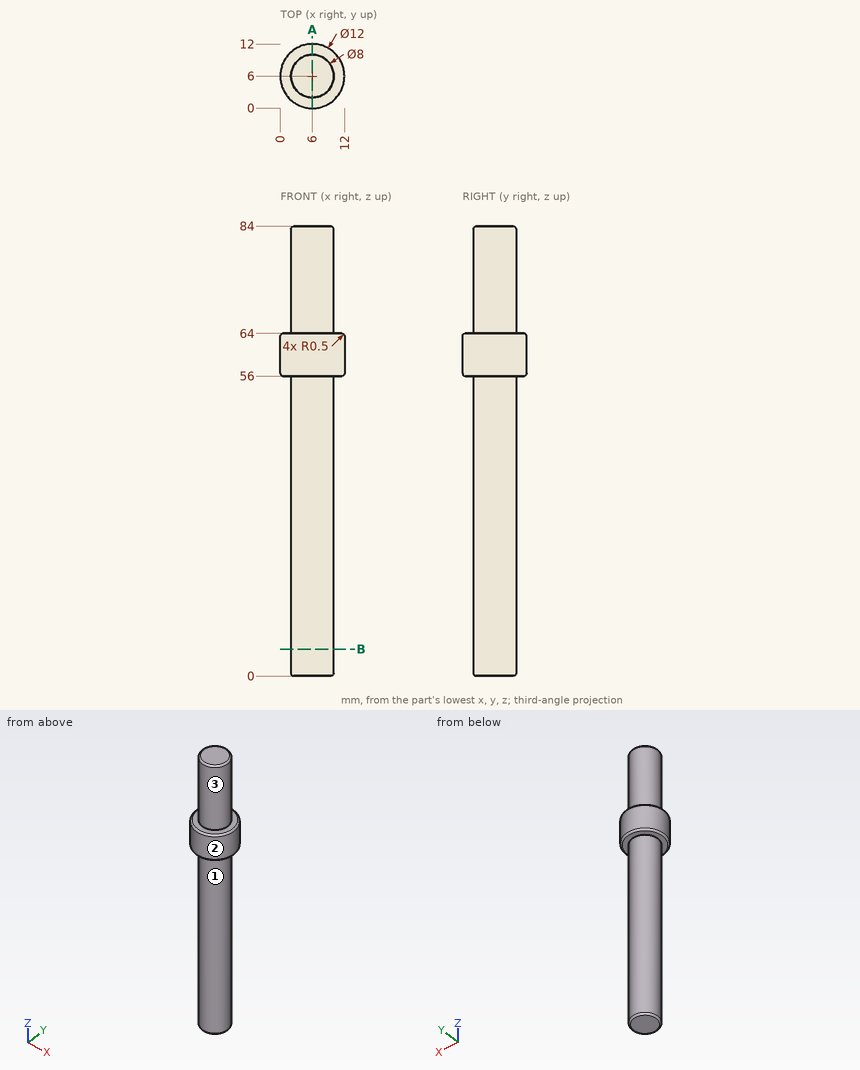
For this review, use the dimensioned drawing (mm, ordinates from the lowest corner) and the shaded views. A direction names the side the tool comes from. Give positions to 0.01 mm unless a question says otherwise; leave off trailing zeros. Order: outer loops, then holes, each group sorted by start corner. A loop starts at its lowest first (then second) coordinate and runs counter-clockwise, first axis right, second up.
1) Take a section at A-A (x = 6). Give the boundary of the cut face in (y, z), then the cut area to 3 significant figures.
2) Insertion check: pin 1 (5 mm diameter, centred on y = 6.5, z = 48, fed in from -X); pin 2 (2 mm diameter, centred on y = 10.5, z = 30, fed in from -X); pin 3 (4 mm diameter, centred on y = 1.5, z = 20, fed in from +X). Each pin has a flat end and moves straight along its axis. Give the tip position at first contact, or say it passes through.
3) Take a section at B-B (z = 5). Give the boundary of the cut face in (x, y).
4) For the marked faces 1, 2 and 3, list the 3-axis set-ups (+Z, -Z, +X, -X, +Y, -Y) from which the entire face can be reached by the end or side of a thin tool; tool diameter is ignored.
5) Wall thickness on line 1 (Z direction, x = 10.5, y = 4.25); line 2 (Z direction, x = 4, y = 3); line 3 (Y direction, x = 6, z = 74.5): over which ranges is each line inside the solid? List them lowest first.
Derived:
1. outline: (0, 56.5) arc R0.5 ccw to (0.5, 56) - (2, 56) - (2, 0.5) arc R0.5 ccw to (2.5, 0) - (9.5, 0) arc R0.5 ccw to (10, 0.5) - (10, 56) - (11.5, 56) arc R0.5 ccw to (12, 56.5) - (12, 63.5) arc R0.5 ccw to (11.5, 64) - (10, 64) - (10, 83.5) arc R0.5 ccw to (9.5, 84) - (2.5, 84) arc R0.5 ccw to (2, 83.5) - (2, 64) - (0.5, 64) arc R0.5 ccw to (0, 63.5) - close
1. area: 704 mm2
2. pin 1: stops at x = 2
2. pin 2: stops at x = 4.06
2. pin 3: stops at x = 9.12
3. outline: circle Ø8 at (6, 6)
4. face 1: -Z
4. face 2: +Z, -Z
4. face 3: +Z
5. line 1: z = 56 to 64
5. line 2: z = 0.01 to 83.99
5. line 3: y = 2 to 10
